Input: part model. Units: mm. Frame: model coordinates. Face numbers are marked on the shaded views. Give positions to 0.01 mm unless a question says otherwise; leave off trailing zeros. Write each loop counter-clockwise with the first axis right and the second up, starting at its lowest first coordinate (ties: lowest second). Pieces come first, ordered by that corner, then holes. Notation, with made-up numbers: (14.5, -31) - (53.5, -31) arc R27 ccw to (53.5, 2) - close; hole circle Ø11 at (69.5, -25). An arc over 180 degrees is marked (long way). Use a Markdown table: item, result. Add a question column.
1. Mould query, pull axis X, two halves, no side actions, for the marked faces 1 and 2. Classes: released by +X, released by -X, zero draft, split by the parting line, or undercut.
2. Section query A-A, the plane z = 0. Return loops of the section in (x, y).
3. Section query D-D, the plane y = -1.25. Count the separate pieces of the cut face and the enclosed holes in it, plus the area to 3 significant figures.
4. Pin query (flat end, axial travel): pin 1 (7 mm diameter, centred on x = -48.16, z = 20, fed in from -Y); pin 2 (4 mm diameter, centred on x = 11.84, z = -15, fed in from +Y); pin 3 (5.5 mm diameter, centred on x = 11.84, z = 15, fed in from -Y). Return the tip coordinate at first contact, or that it passes through.
5. Section query B-B, the plane y = -6.75. Return loops of the section in (x, z) (3 decimals).
6. Section query C-C, the plane z = -10.5. Return loops of the section in (x, y).
7. Material intervals for probe 1 along Z at (x, y) = (-44, -7.5); probe 2 along X at (y, z) = (-2.5, 17.5); probe 3 along Z at (x, y) = (-6.5, -5.75), sorted ascending.
```python
from build123d import *

# Parameters (mm, degrees)
F0_W           = 116
F0_H           = 60
F1_DEPTH       = 8
F3_D           = 5.5
F3_DEPTH       = 13.8
F3_CBORE_D     = 9.75
F3_CBORE_DEPTH = 5
F3_TIP         = 1.6523667023
F4_D           = 16
F4_DEPTH       = 13.8
F4_CBORE_D     = 40
F4_CBORE_DEPTH = 3.5
F4_TIP         = 4.8068849522
F5_D           = 3.3
F5_DEPTH       = 13.8
F5_CBORE_D     = 6.5
F5_CBORE_DEPTH = 3
F5_TIP         = 0.9914200214


with BuildPart() as f1:
    # F0 (on Front) → F1 (new body)
    with BuildSketch(Plane.XZ):
        with Locations((1.8354473706, 0.0017675648)):
            Rectangle(F0_W, F0_H)
    extrude(amount=F1_DEPTH)

    # F3
    with Locations(Plane.XZ.offset(8)):
        with Locations((-48.1645526294, 20.0017675648), (-48.1645526294, -19.9982324352), (51.8354473706, 20.0017675648), (51.8354473706, -19.9982324352)):
            CounterBoreHole(F3_D / 2, F3_CBORE_D / 2, F3_CBORE_DEPTH, depth=F3_DEPTH)
            with Locations((0, 0, -(F3_DEPTH + F3_TIP / 2))):  # 118° drill point
                Cone(0, F3_D / 2, F3_TIP, mode=Mode.SUBTRACT)

    # F4
    with Locations(Plane.XZ.offset(8)):
        with Locations((11.8354473706, 0)):
            CounterBoreHole(F4_D / 2, F4_CBORE_D / 2, F4_CBORE_DEPTH, depth=F4_DEPTH)
            with Locations((0, 0, -(F4_DEPTH + F4_TIP / 2))):  # 118° drill point
                Cone(0, F4_D / 2, F4_TIP, mode=Mode.SUBTRACT)

    # F5
    with Locations(Plane(origin=(0, 0, 0), x_dir=(1, 0, 0), z_dir=(0, 1, 0))):
        with Locations((11.8354473706, -15), (26.8354473706, 0), (11.8354473706, 15), (-3.1645526294, 0)):
            CounterBoreHole(F5_D / 2, F5_CBORE_D / 2, F5_CBORE_DEPTH, depth=F5_DEPTH)
            with Locations((0, 0, -(F5_DEPTH + F5_TIP / 2))):  # 118° drill point
                Cone(0, F5_D / 2, F5_TIP, mode=Mode.SUBTRACT)


solid = f1.part
```
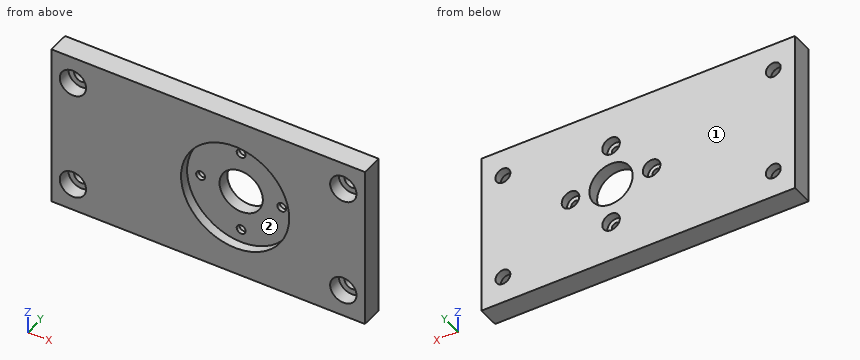
Result sheet:
| question | item | result |
|---|---|---|
| 1 | face 1 | zero draft |
| 1 | face 2 | undercut |
| 2 | outline | (-56.16, -8) - (-8.16, -8) - (-8.16, -4.5) - (-4.81, -4.5) - (-4.81, -3) - (-6.41, -3) - (-6.41, 0) - (-56.16, 0) - close; (-1.51, -4.5) - (3.84, -4.5) - (3.84, 0) - (0.09, 0) - (0.09, -3) - (-1.51, -3) - close; (19.84, -4.5) - (25.19, -4.5) - (25.19, -3) - (23.59, -3) - (23.59, 0) - (19.84, 0) - close; (28.49, -4.5) - (31.84, -4.5) - (31.84, -8) - (59.84, -8) - (59.84, 0) - (30.09, 0) - (30.09, -3) - (28.49, -3) - close |
| 3 | separate pieces | 1 |
| 3 | enclosed holes | 9 |
| 3 | area | 6,530 mm² |
| 4 | pin 1 | stops at y = -3 |
| 4 | pin 2 | stops at y = -3 |
| 4 | pin 3 | stops at y = -4.5 |
| 5 | outline | (-56.165, -29.998) - (59.835, -29.998) - (59.835, 30.002) - (-56.165, 30.002) - close; hole circle Ø9.75 at (-48.165, -19.998); hole circle Ø9.75 at (-48.165, 20.002); hole circle Ø40 at (11.835, 0); hole circle Ø9.75 at (51.835, -19.998); hole circle Ø9.75 at (51.835, 20.002) |
| 6 | outline | (-56.16, -8) - (-5.19, -8) - (-5.19, -4.5) - (28.86, -4.5) - (28.86, -8) - (59.84, -8) - (59.84, 0) - (-56.16, 0) - close |
| 7 | probe 1 | z = -30 to -22.53, -17.46 to 17.47, 22.54 to 30 |
| 7 | probe 2 | x = -56.16 to -49.31, -47.02 to 9.76, 13.91 to 50.69, 52.98 to 59.84 |
| 7 | probe 3 | z = -30 to -7.99, 7.99 to 30 |
